```python
from build123d import *

# Parameters (mm, degrees)
SKETCH1_W           = 42.4
SKETCH1_H           = 42.4
BOSS_EXTRUDE1_DEPTH = 49
SKETCH2_R           = 11.25
BOSS_EXTRUDE2_DEPTH = 2
SKETCH3_R           = 2.5
BOSS_EXTRUDE3_DEPTH = 22.5


with BuildPart() as part:
    # Sketch1 → Boss-Extrude1 (new body)
    with BuildSketch(Plane.XY):
        with Locations((-4.195833333, 4.30625)):
            Rectangle(SKETCH1_W, SKETCH1_H)
    extrude(amount=BOSS_EXTRUDE1_DEPTH)

    # Sketch2 → Boss-Extrude2 (add)
    with BuildSketch(Plane.XY.offset(49)):
        with Locations((-4.195833333, 4.30625)):
            Circle(SKETCH2_R)
    extrude(amount=BOSS_EXTRUDE2_DEPTH)

    # Sketch3 → Boss-Extrude3 (add)
    with BuildSketch(Plane.XY.offset(51)):
        with Locations(Location((-4.195833333, 4.30625, 0), (0, 0, 180))):
            Circle(SKETCH3_R)
    extrude(amount=BOSS_EXTRUDE3_DEPTH)


solid = part.part
```
Could you check a few things on this model? Use its own coordinates, in mm. A direction names the side the tool comes from. Round coordinates to 2 decimals unless told otherwise and drop trailing zeros. Loops run counter-clockwise (first coordinate to the right, second up) from the corner with the lowest first, then second, coordinate; pieces in that order, holes last.
Q1. I want a section at B-B (x = -10). Write out the boundary of the cut face in (y, z).
Q2. I want a section at A-A (y = -3.5). Write out the boundary of the cut face in (x, z), and give its area (3 significant figures).
Q3. On a 3-axis mill with a long thin cutter (end or side, diameter ignored), from which of +Z, -Z, +X, -X, +Y, -Y can I reach the whole of each face in a straight line? I mean faces 1 (the cylindrical face through (-6.635, -6.676, 49.986)), 2 (the flat face through (-4, -16.894, 24)). Say none if no direction works.
Q4. I want a section at C-C (y = 18). Write out the boundary of the cut face in (x, z).
Q5. I want a section at D-D (z = 50). Write out the boundary of the cut face in (x, y).
Q6. Please list where these lines run through material, in increasing order: L1, parallel to Z at x = 13, y = 15; L2, parallel to Z at x = -6, y = 15; L3, parallel to X at y = 3, z = 57.5.
Answer below:
1. outline: (-16.89, 0) - (25.51, 0) - (25.51, 49) - (13.94, 49) - (13.94, 51) - (-5.33, 51) - (-5.33, 49) - (-16.89, 49) - close
2. outline: (-25.4, 0) - (17, 0) - (17, 49) - (3.91, 49) - (3.91, 51) - (-12.3, 51) - (-12.3, 49) - (-25.4, 49) - close
2. area: 2,110 mm2
3. face 1: +Z
3. face 2: +Z, -Z, +X, -X, -Y
4. outline: (-25.4, 0) - (17, 0) - (17, 49) - (-25.4, 49) - close
5. outline: circle Ø22.5 at (-4.2, 4.31)
6. L1: z = 0 to 49
6. L2: z = 0 to 51
6. L3: x = -6.33 to -2.06
